Geometry: final body of the model. Coordinates: model frame, mm. Face numbers are marked on the shaded views. A direction names the side the tool comes from. Round coordinates to 2 decimals unless told otherwise and drop trailing zeros. Loops run counter-clockwise (first coordinate to the right, second up) from the corner with the lowest first, then second, coordinate; pieces in that order, holes last. Notation, with made-up numbers: M 47.5,48 L 86.5,48 A31 ccw 86.5,86 Z; hole C -14.75,0.25 d10. An arc over 180 degrees is marked long. Answer as a JSON object with one key per item and string values.
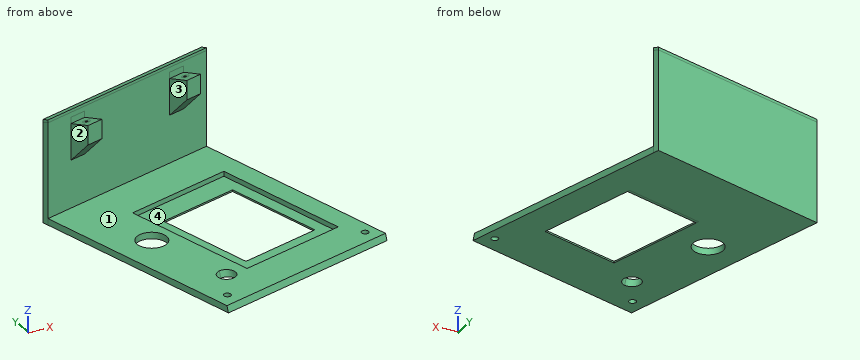
from build123d import *

# Parameters (mm, degrees)
SALIENTE_EXTRUIR1_START       = 2.11e-07
SALIENTE_EXTRUIR1_DEPTH       = 36.2755111
SALIENTE_EXTRUIR1_START_2     = 19.300740439
SALIENTE_EXTRUIR1_2_DEPTH     = 15.222231072
SALIENTE_EXTRUIR1_3_DEPTH     = 0.575969357
SALIENTE_EXTRUIR1_START_3     = 0.575969568
SALIENTE_EXTRUIR1_4_DEPTH     = 1.75
SALIENTE_EXTRUIR1_START_4     = -30.997891642
SALIENTE_EXTRUIR1_5_DEPTH     = 69
SALIENTE_EXTRUIR1_6_OUTLINE_W = 15.703224266
SALIENTE_EXTRUIR1_6_OUTLINE_H = 2.325969357
SALIENTE_EXTRUIR1_6_DEPTH     = 69
SALIENTE_EXTRUIR1_7_DEPTH     = 21.66081402
SALIENTE_EXTRUIR1_START_5     = 30.341294328
SALIENTE_EXTRUIR1_8_DEPTH     = 7.66081403
SALIENTE_EXTRUIR2_DEPTH       = 1
CROQUIS3_R                    = 1.25
CORTAR_EXTRUIR1_DEPTH         = 10
CROQUIS4_R                    = 5.324975084
CORTAR_EXTRUIR2_DEPTH         = 10
SALIENTE_EXTRUIR3_DEPTH       = 69
CORTAR_EXTRUIR3_DEPTH         = 69
SALIENTE_EXTRUIR4_REACH       = 101.278
CROQUIS7_R                    = 1.25
CROQUIS7_R_2                  = 0.5


with BuildPart() as part:
    # Saliente-Extruir1: read off the stored shape, not the designer's step
    # Saliente-Extruir1 outline → Saliente-Extruir1 (new body)
    with BuildSketch(Plane.XY.offset(SALIENTE_EXTRUIR1_START)):
        Polygon((-51.625046866, 66.023279607), (-50.996835351, 63.877170392), (15.224363662, 83.261514624), (14.596152147, 85.407623839), align=None)
    extrude(amount=SALIENTE_EXTRUIR1_DEPTH)

    # Saliente-Extruir1 2 outline → Saliente-Extruir1 2 (add)
    with BuildSketch(Plane.XY.offset(SALIENTE_EXTRUIR1_START_2)):
        Polygon((-35.641195, 68.372090794), (-41.399560131, 66.686495643), (-39.242610722, 59.317880312), (-33.484245591, 61.003475463), align=None)
        Polygon((5.627088443, 80.452189373), (-0.131276689, 78.766594222), (2.02567272, 71.397978892), (7.784037852, 73.083574042), align=None)
    extrude(amount=SALIENTE_EXTRUIR1_2_DEPTH)

    # Saliente-Extruir1 3 outline → Saliente-Extruir1 3 (add)
    # profile 1 of 3: a face of its own
    with BuildSketch(Plane.XY.offset(SALIENTE_EXTRUIR1_START)):
        Polygon((-35.641195, 68.372090794), (-41.399560131, 66.686495643), (-39.242610722, 59.317880312), (-33.484245591, 61.003475463), align=None)
    # profile 2 of 3: a face of its own
    with BuildSketch(Plane.XY.offset(SALIENTE_EXTRUIR1_START)):
        Polygon((5.627088443, 80.452189373), (-0.131276689, 78.766594222), (2.02567272, 71.397978892), (7.784037852, 73.083574042), align=None)
    # profile 3 of 3: a face of its own
    with BuildSketch(Plane.XY.offset(SALIENTE_EXTRUIR1_START)):
        Polygon((-25.796809543, 54.891581059), (-11.360360521, 5.573484337), (26.720065065, 16.720429561), (12.283616043, 66.038526283), align=None)
        Polygon((-18.597227896, 49.301446301), (10.194597762, 57.729422054), (20.870033716, 21.259776221), (-7.921791942, 12.831800468), align=None, mode=Mode.SUBTRACT)
    extrude(amount=SALIENTE_EXTRUIR1_3_DEPTH)

    # Saliente-Extruir1 4 outline → Saliente-Extruir1 4 (add)
    with BuildSketch(Plane.XY.offset(SALIENTE_EXTRUIR1_START_3)):
        Polygon((-35.641195, 68.372090794), (-41.399560131, 66.686495643), (-39.242610722, 59.317880312), (-33.484245591, 61.003475463), align=None)
        Polygon((5.627088443, 80.452189373), (-0.131276689, 78.766594222), (2.02567272, 71.397978892), (7.784037852, 73.083574042), align=None)
    extrude(amount=SALIENTE_EXTRUIR1_4_DEPTH)

    # Saliente-Extruir1 5 outline → Saliente-Extruir1 5 (cut)
    with BuildSketch(Plane(origin=(0, 0, 0), x_dir=(-0.2809325251095079, 0.9597275219225484, 0), z_dir=(0.9597275219225485, 0.2809325251095079, 0)).offset(SALIENTE_EXTRUIR1_START_4)):
        Polygon((67.953527999, 19.300740439), (75.631348175, 19.300740439), (67.953528, 27.634470761), align=None)
        Polygon((67.953528, 34.522971511), (75.631348175, 32.275511311), (75.631348175, 34.522971511), align=None)
        Polygon((75.631348175, 36.275511311), (77.867513301, 35.620938527), (77.867513301, 36.275511311), align=None)
    extrude(amount=SALIENTE_EXTRUIR1_5_DEPTH, mode=Mode.SUBTRACT)

    # Saliente-Extruir1 6 outline → Saliente-Extruir1 6 (add)
    with BuildSketch(Plane(origin=(0, 0, 0), x_dir=(-0.2809325251095079, 0.9597275219225484, 0), z_dir=(0.9597275219225485, 0.2809325251095079, 0)).offset(SALIENTE_EXTRUIR1_START_4)):
        with Locations((67.779736042, 1.16298489)):
            Rectangle(SALIENTE_EXTRUIR1_6_OUTLINE_W, SALIENTE_EXTRUIR1_6_OUTLINE_H)
        Polygon((8.540521078, 2.11e-07), (8.540521079, 2.325969568), (-5.302071851, 2.325969568), (-5.982932231, 2.11e-07), align=None)
    extrude(amount=SALIENTE_EXTRUIR1_6_DEPTH)

    # Saliente-Extruir1 7 outline → Saliente-Extruir1 7 (add)
    with BuildSketch(Plane(origin=(0, 0, 0), x_dir=(-0.2809325251095079, 0.9597275219225484, 0), z_dir=(0.9597275219225485, 0.2809325251095079, 0)).offset(SALIENTE_EXTRUIR1_START_4)):
        Polygon((59.928123909, 2.11e-07), (59.928123909, 2.325969568), (8.540521079, 2.325969568), (8.540521078, 2.11e-07), align=None)
    extrude(amount=SALIENTE_EXTRUIR1_7_DEPTH)

    # Saliente-Extruir1 8 outline → Saliente-Extruir1 8 (add)
    with BuildSketch(Plane(origin=(0, 0, 0), x_dir=(-0.2809325251095079, 0.9597275219225484, 0), z_dir=(0.9597275219225485, 0.2809325251095079, 0)).offset(SALIENTE_EXTRUIR1_START_5)):
        Polygon((59.928123909, 2.11e-07), (59.928123909, 2.325969568), (8.540521079, 2.325969568), (8.540521078, 2.11e-07), align=None)
    extrude(amount=SALIENTE_EXTRUIR1_8_DEPTH)

    # Saliente-Extruir1 9: loft between two sections, ruled curve by curve
    saliente_extruir1_9_from = [
        Edge.make_bspline([(-17.960997328, 1.936811392, 2.325969568), (-24.199226221, 0.110749979, 2.325969568), (-26.025287634, 6.348978871, 2.325969568), (-19.787058741, 8.175040285, 2.325969568)], [0, 0, 0, 0, 1, 1, 1, 1], 3, [1, 0.333333333, 0.333333333, 1]),
        Edge.make_bspline([(-19.787058741, 8.175040285, 2.325969568), (-13.548829849, 10.001101698, 2.325969568), (-11.722768436, 3.762872805, 2.325969568), (-17.960997328, 1.936811392, 2.325969568)], [0, 0, 0, 0, 1, 1, 1, 1], 3, [1, 0.333333333, 0.333333333, 1]),
    ]
    saliente_extruir1_9_to = [
        Edge.make_bspline([(-17.769721503, 1.283370947, 2.11e-07), (-24.007950395, -0.542690466, 2.11e-07), (-25.834011808, 5.695538426, 2.11e-07), (-19.595782916, 7.52159984, 2.11e-07)], [0, 0, 0, 0, 1, 1, 1, 1], 3, [1, 0.333333333, 0.333333333, 1]),
        Edge.make_bspline([(-19.595782916, 7.52159984, 2.11e-07), (-13.357554023, 9.347661253, 2.11e-07), (-11.53149261, 3.10943236, 2.11e-07), (-17.769721503, 1.283370947, 2.11e-07)], [0, 0, 0, 0, 1, 1, 1, 1], 3, [1, 0.333333333, 0.333333333, 1]),
    ]
    saliente_extruir1_9 = Solid(Shell([*[Face.make_surface_from_curves(saliente_extruir1_9_from[k], saliente_extruir1_9_to[k]) for k in range(2)], Face(Wire(saliente_extruir1_9_from)), Face(Wire(saliente_extruir1_9_to))]))
    add(saliente_extruir1_9, mode=Mode.SUBTRACT)

    # Saliente-Extruir1 10: loft between two sections, ruled curve by curve
    saliente_extruir1_10_from = [
        Edge.make_three_point_arc((5.262809235, 75.46739376, 30.520058845), (3.726126487, 76.267574249, 30.168893189), (2.86349043, 74.765062447, 30.520058845)),
        Edge.make_three_point_arc((2.86349043, 74.765062447, 30.520058845), (4.400173178, 73.964881958, 30.871224502), (5.262809235, 75.46739376, 30.520058845)),
    ]
    saliente_extruir1_10_to = [
        Edge.make_three_point_arc((5.026039984, 76.276249789, 33.399241411), (3.489357236, 77.076430278, 33.048075755), (2.626721179, 75.573918476, 33.399241411)),
        Edge.make_three_point_arc((2.626721179, 75.573918476, 33.399241411), (4.163403927, 74.773737987, 33.750407067), (5.026039984, 76.276249789, 33.399241411)),
    ]
    saliente_extruir1_10 = Solid(Shell([*[Face.make_surface_from_curves(saliente_extruir1_10_from[k], saliente_extruir1_10_to[k]) for k in range(2)], Face(Wire(saliente_extruir1_10_from)), Face(Wire(saliente_extruir1_10_to))]))
    add(saliente_extruir1_10, mode=Mode.SUBTRACT)

    # Saliente-Extruir1 11: loft between two sections, ruled curve by curve
    saliente_extruir1_11_from = [
        Edge.make_three_point_arc((-36.868110265, 61.884783379, 30.871224502), (-36.005474208, 63.387295181, 30.520058845), (-37.542156955, 64.18747567, 30.168893189)),
        Edge.make_three_point_arc((-37.542156955, 64.18747567, 30.168893189), (-38.404793012, 62.684963868, 30.520058845), (-36.868110265, 61.884783379, 30.871224502)),
    ]
    saliente_extruir1_11_to = [
        Edge.make_three_point_arc((-37.104879516, 62.693639407, 33.750407067), (-36.242243459, 64.196151209, 33.399241411), (-37.778926206, 64.996331698, 33.048075755)),
        Edge.make_three_point_arc((-37.778926206, 64.996331698, 33.048075755), (-38.641562263, 63.493819896, 33.399241411), (-37.104879516, 62.693639407, 33.750407067)),
    ]
    saliente_extruir1_11 = Solid(Shell([*[Face.make_surface_from_curves(saliente_extruir1_11_from[k], saliente_extruir1_11_to[k]) for k in range(2)], Face(Wire(saliente_extruir1_11_from)), Face(Wire(saliente_extruir1_11_to))]))
    add(saliente_extruir1_11, mode=Mode.SUBTRACT)

    # Saliente-Extruir1 12: loft between two sections, ruled curve by curve
    saliente_extruir1_12_from = [
        Edge.make_three_point_arc((-30.979047738, 39.986658971, 2.325969568), (-25.396077527, 36.932081486, 2.325969568), (-28.450655012, 31.349111274, 2.325969568)),
        Edge.make_three_point_arc((-28.450655012, 31.349111274, 2.325969568), (-34.033625224, 34.40368876, 2.325969568), (-30.979047738, 39.986658971, 2.325969568)),
    ]
    saliente_extruir1_12_to = [
        Edge.make_three_point_arc((-30.979047738, 39.986658971, 2.11e-07), (-25.396077527, 36.932081486, 2.11e-07), (-28.450655012, 31.349111274, 2.11e-07)),
        Edge.make_three_point_arc((-28.450655012, 31.349111274, 2.11e-07), (-34.033625224, 34.40368876, 2.11e-07), (-30.979047738, 39.986658971, 2.11e-07)),
    ]
    saliente_extruir1_12 = Solid(Shell([*[Face.make_surface_from_curves(saliente_extruir1_12_from[k], saliente_extruir1_12_to[k]) for k in range(2)], Face(Wire(saliente_extruir1_12_from)), Face(Wire(saliente_extruir1_12_to))]))
    add(saliente_extruir1_12, mode=Mode.SUBTRACT)

    # Croquis2 → Saliente-Extruir2 (add)
    with BuildSketch(Plane(origin=(-14.760341257, 50.424584095, 0), x_dir=(-0.9597275219225485, -0.28093252510950767, 0), z_dir=(0.28093252510950767, -0.9597275219225485, 0))):
        Polygon((3.997891642, -0.575969568), (-26.002108358, -0.575969568), (-26.002108358, -2.11e-07), (3.997891642, 0), align=None)
    extrude(amount=SALIENTE_EXTRUIR2_DEPTH)

    # Croquis3 → Cortar-Extruir1 (cut)
    with BuildSketch(Plane.XY.offset(2.325969568)):
        with Locations((32.57715474, 9.742255252)):
            Circle(CROQUIS3_R)
        with Locations((-24.975865422, -7.104729869)):
            Circle(CROQUIS3_R)
    extrude(amount=-CORTAR_EXTRUIR1_DEPTH, mode=Mode.SUBTRACT)

    # Croquis4 → Cortar-Extruir2 (cut)
    with BuildSketch(Plane(origin=(0, 0, 0), x_dir=(-1, 0, 0), z_dir=(0, 0, -1))):
        with Locations(Location((28.971074723, 36.024788725, 0), (0, 0, 90))):
            Circle(CROQUIS4_R)
    extrude(amount=-CORTAR_EXTRUIR2_DEPTH, mode=Mode.SUBTRACT)

    # Croquis5 → Saliente-Extruir3 (add)
    with BuildSketch(Plane(origin=(36.471669282, 10.67602826, 0), x_dir=(0, 0, -1), z_dir=(0.9597275219225486, 0.28093252510950756, 0))):
        Polygon((-36.275511311, 75.631348175), (-37.275511311, 75.631348175), (-36.620938527, 77.867513301), (-35.620938527, 77.867513301), align=None)
    extrude(amount=-SALIENTE_EXTRUIR3_DEPTH)

    # Croquis6 → Cortar-Extruir3 (cut)
    with BuildSketch(Plane(origin=(36.471669282, 10.67602826, 0), x_dir=(0, 0, -1), z_dir=(0.9597275219225486, 0.28093252510950756, 0))):
        Polygon((-2.325969568, -5.302071851), (-2.325969568, -4.802071851), (-2.11e-07, -5.482932231), (-2.11e-07, -5.982932231), align=None)
    extrude(amount=-CORTAR_EXTRUIR3_DEPTH, mode=Mode.SUBTRACT)

    # Croquis7 → Saliente-Extruir4 (add, up to next)
    with BuildSketch(Plane(origin=(-4.121600365, 14.080296693, 50.119852402), x_dir=(0.9968807084425405, 0.021345720862208265, 0.07598166447223464), z_dir=(-0.07892308366440427, 0.2696186761507921, 0.9597275219225484)), mode=Mode.PRIVATE) as saliente_extruir4_sk1:
        with Locations((-33.424563455, 52.432282093)):
            Circle(CROQUIS7_R)
        with Locations(Location((-33.424563455, 52.432282093, 0), (0, 0, 270.000000004))):
            Circle(CROQUIS7_R_2, mode=Mode.SUBTRACT)
    saliente_extruir4_tool1 = extrude(saliente_extruir4_sk1.sketch, amount=-SALIENTE_EXTRUIR4_REACH, mode=Mode.PRIVATE) - part.part
    # Croquis7 → Saliente-Extruir4 (add, up to next)
    with BuildSketch(Plane(origin=(-4.121600365, 14.080296693, 50.119852402), x_dir=(0.9968807084425405, 0.021345720862208265, 0.07598166447223464), z_dir=(-0.07892308366440427, 0.2696186761507921, 0.9597275219225484)), mode=Mode.PRIVATE) as saliente_extruir4_sk2:
        with Locations((7.972850592, 64.062162154)):
            Circle(CROQUIS7_R)
        with Locations(Location((7.972850592, 64.062162154, 0), (0, 0, 270.000000007))):
            Circle(CROQUIS7_R_2, mode=Mode.SUBTRACT)
    saliente_extruir4_tool2 = extrude(saliente_extruir4_sk2.sketch, amount=-SALIENTE_EXTRUIR4_REACH, mode=Mode.PRIVATE) - part.part
    add(saliente_extruir4_tool1.solids().sort_by_distance((-38.652759, 63.819058, 33.306951))[0])
    add(saliente_extruir4_tool2.solids().sort_by_distance((2.615525, 75.899157, 33.306951))[0])


solid = part.part
1) Section query B-B (z = 22.5). Return the cut outline in (x, y).
Results:
{"outline": "M -51.63,66.02 L -51,63.88 L -41.4,66.69 L -40.57,63.86 L -34.81,65.54 L -35.64,68.37 L -0.13,78.77 L 0.7,75.94 L 6.46,77.62 L 5.63,80.45 L 15.22,83.26 L 14.6,85.41 Z"}
2) Section query A-A (y = 15). Return the cut outline in (x, z).
Results:
{"outline": "M -36.69,0 L -8.56,0 L -8.56,0.58 L -14.12,0.58 L -14.12,2.33 L -36.69,2.33 Z; M -0.51,0 L 35.21,0 L 35.21,2.33 L 20.84,2.33 L 20.84,0.58 L -0.51,0.58 Z"}
3) Section query D-D (y = -0.5). Return the cut outline in (x, z).
Results:
{"outline": "M -32.15,0 L 17.81,0 L 15.39,2.33 L -32.15,2.33 Z"}
4) Ray query, line 1 (Z direction, x = 15.5, y = 15.5); line 2 (Z direction, x = 26.5, y = 37.5); line 3 (Y direction, x = -2.5, z = 27). Return the intervals inside material, ascending.
Results:
{"line 1": "0 to 0.58", "line 2": "0 to 2.33", "line 3": "78.07 to 80.4"}
5) Pin query (flat end, axial travel): P1, Ø10, axis at x = -13.5, z = 6.5, coming from the -Y side; P2, Ø1.5, axis at x = -31.5, z = 23.5, coming from the +Y side; P3, Ø16, axis at x = 2, y = 40.5, coming from the +Z side; P4, Ø1, axis at x = -9.5, y = 67.5, coming from the +Z side. Return the tip coordinate at first contact, or that it passes through.
Results:
{"P1": "y = -9.76", "P2": "y = 72.13", "P3": "through", "P4": "z = 2.33"}
6) Section query C-C (x = 24). Return the cut outline in (y, z), and give its area (3 significant figures).
Results:
{"outline": "M 1.31,0 L 53.28,0 L 53.28,2.33 L 26.01,2.33 L 26.01,0.58 L 15.92,0.58 L 15.92,2.33 L 2.02,2.33 Z", "area": "102 mm2"}
7) Pull-direction query (X, two-part tool) for the marked faces 1 and 2; classes: +X half, -X half, draft (parallel to the pull), parting line (faces both ways), or undercut.
Results:
{"face 1": "draft", "face 2": "undercut"}
8) Reachability of the marked faces 3 and 4 from +Z, -Z, +X, -X, +Y, -Y: full face, straight path, thin tool, end or side. Return the list, or none.
Results:
{"face 3": "+Z, -Y", "face 4": "+Z"}
